Geometry: final body of the model. Coordinates: model frame, mm. Coordinates: 2 decimals unless noted, no trailing zeros. Write each loop counter-clockwise with the first axis right and the second up, starting at its lowest first coordinate (ties: lowest second). Pieces come first, ordered by that corner, then holes. Notation, with made-up numbers: (-22.75, 0.25) - (11.25, 0.25) arc R11 ccw to (11.25, 7.25) - close; hole circle Ø5 at (2.5, -30). An arc over 180 degrees is marked (long way). Put each result on its own line as item: value.
```python
from build123d import *

# Parameters (mm, degrees)
SKETCH1_W           = 56.55
SKETCH1_H           = 197.425
BOSS_EXTRUDE1_DEPTH = 3.175
SKETCH2_R           = 5
CUT_EXTRUDE1_DEPTH  = 10
LPATTERN1_COUNT     = 6
LPATTERN1_PITCH     = 11
SKETCH5_W           = 3.175
SKETCH5_H           = 197.425
BOSS_EXTRUDE2_DEPTH = 19.525


with BuildPart() as part:
    # Sketch1 → Boss-Extrude1 (new body)
    with BuildSketch(Plane.XY):
        Rectangle(SKETCH1_W, SKETCH1_H)
    extrude(amount=BOSS_EXTRUDE1_DEPTH)

    # Sketch2 → Cut-Extrude1 (cut)
    with BuildSketch(Plane(origin=(0, 0, 0), x_dir=(-1, 0, 0), z_dir=(0, 0, -1))):
        with Locations((11.5, -57.369162839)):
            Circle(SKETCH2_R)
        with Locations((-11.5, -57.369162839)):
            Circle(SKETCH2_R)
        with Locations((11.5, 18.830837161)):
            Circle(SKETCH2_R)
        with Locations((0, 18.830837161)):
            Circle(SKETCH2_R)
        with Locations((-11.5, 18.830837161)):
            Circle(SKETCH2_R)
        with Locations((0, -57.369162839)):
            Circle(SKETCH2_R)
    cut_extrude1 = extrude(amount=-CUT_EXTRUDE1_DEPTH, mode=Mode.SUBTRACT)

    # LPattern1: Cut-Extrude1 ×6
    with Locations(*[(0, i * LPATTERN1_PITCH, 0) for i in range(1, LPATTERN1_COUNT)]):
        add(cut_extrude1, mode=Mode.SUBTRACT)

    # Sketch5 → Boss-Extrude2 (add)
    with BuildSketch(Plane.ZY.offset(28.275)):
        with Locations((1.5875, 0)):
            Rectangle(SKETCH5_W, SKETCH5_H)
    extrude(amount=BOSS_EXTRUDE2_DEPTH)


solid = part.part
```
1. Section query B-B (x = 11.5). Count the separate pieces of the cut face and the enclosed holes in it, then the cut area to 3 significant figures.
Answer below:
separate pieces: 13
enclosed holes: 0
area: 246 mm²
2. Ray query, probe 1 along X at (y, z) = (-36, 0.8) (3 decimals); probe 2 along X at (y, z) = (55, 2.3) (3 decimals). Return the intervals inside material, ascending. Write a range as from..to.
Answer below:
probe 1: x = -47.8..-16.46, -6.54..-4.96, 4.96..6.54, 16.46..28.275
probe 2: x = -47.8..-15.367, -7.633..-3.867, 3.867..7.633, 15.367..28.275
3. Mould query, pull axis Y, two halves, no side actions, for faces 1 (the cylindrical face through (-14.188, -53.153, 1.565)), 2 (the flat face through (-47.8, 1, 2)), 3 (the flat face through (-9, 98.712, 2)). Classes: +Y half, -Y half, draft (parallel to the pull), parting line (faces both ways), or undercut.
Answer below:
face 1: undercut
face 2: draft
face 3: +Y half
4. Pin query (flat end, axial travel): pin 1 Ø12 at (x, y) = (-4.5, 13) entering from -Z; pin 2 Ø8 at (x, y) = (11.5, 62.83) entering from +Z. Return the tip coordinate at first contact, or that it passes through.
Answer below:
pin 1: stops at z = 0
pin 2: passes through
5. Section query A-A (y = 49). Return loops of the section in (x, z) (3 decimals), then the cut area to 3 significant figures.
Answer below:
outline: (-47.8, 0) - (-15.621, 0) - (-15.621, 3.175) - (-47.8, 3.175) - close; (-7.379, 0) - (-4.121, 0) - (-4.121, 3.175) - (-7.379, 3.175) - close; (4.121, 0) - (7.379, 0) - (7.379, 3.175) - (4.121, 3.175) - close; (15.621, 0) - (28.275, 0) - (28.275, 3.175) - (15.621, 3.175) - close
area: 163 mm²
